Design review of the part built by this model. Coordinates are the model's own, in mm. A direction names the side the tool comes from. Give positions to 0.01 mm unless a question says otherwise; leave off trailing zeros. Order: outer loops, then holes, each group sorted by start corner. A loop starts at its lowest first (then second) coordinate and runs counter-clockwise, first axis right, second up. Notation, with made-up numbers: M 13.25,67 L 60.25,67 A15 cw 60.25,88 Z; hole C 60,40 d9. An arc over 180 degrees is marked long. Answer as a JSON object with one key per item and string values.
from build123d import *

# Parameters (mm, degrees)
SKETCH3_R          = 2.2
CUT_EXTRUDE1_DEPTH = 150


with BuildPart() as part:
    # Sketch1 → Revolve1 (revolve)
    with BuildSketch(Plane.XY, mode=Mode.PRIVATE) as revolve1_sk:
        with BuildLine():
            Line((0, 0), (152, 0))
            ThreePointArc((152, 0), (151.747967345, 2.795084972), (151, 5.5))
            Line((151, 5.5), (150, 5.5))
            Line((150, 5.5), (150, 4.5))
            Line((150, 4.5), (141, 4.5))
            Line((141, 4.5), (141, 3.5))
            Line((141, 3.5), (0, 3.5))
            Line((0, 3.5), (0, 0))
        make_face()
    revolve(revolve1_sk.sketch.rotate(Axis((0, 0, 0), (1, 0, 0)), 90), axis=Axis((0, 0, 0), (1, 0, 0)))

    # Sketch2 → Revolve2 (revolve)
    with BuildSketch(Plane.XY, mode=Mode.PRIVATE) as revolve2_sk:
        with BuildLine():
            Line((6, 0), (7, 0))
            Line((7, 0), (7, 3.5))
            ThreePointArc((7, 3.5), (6.5, 3.7), (6, 3.5))
            Line((6, 3.5), (6, 0))
        make_face()
    revolve(revolve2_sk.sketch.rotate(Axis((6, 0, 0), (1, 0, 0)), 90), axis=Axis((6, 0, 0), (1, 0, 0)))

    # Sketch3 → Cut-Extrude1 (cut)
    with BuildSketch(Plane.ZY):
        Circle(SKETCH3_R)
    extrude(amount=-CUT_EXTRUDE1_DEPTH, mode=Mode.SUBTRACT)


solid = part.part
(1) Insertion check: pin 1 (4 mm diameter, centred on x = 129, z = 0.5, fed in from -Y); pin 2 (6 mm diameter, centred on x = 109, z = 4, fed in from +Y); pin 3 (2.5 mm diameter, centred on y = 0, z = 0, fed in from -X). Each pin has a flat end and moves straight along its axis. Give the tip position at first contact, or say it passes through.
Checked values:
{"pin 1": "stops at y = -3.5", "pin 2": "stops at y = 3.35", "pin 3": "stops at x = 150"}
(2) We need section C-C (x = 70). Write out the cut boundary in (y, z).
Checked values:
{"outline": "C 0,0 d7; hole C 0,0 d4.4"}
(3) Draft analysis for pull direction Y (two halves, no side actions). For faces 1 (the cylindrical face through (73.062, 3.105, 1.615)), 2 (the cylindrical face through (73.95, 0.66, 2.1)), 3 (the flat face through (0, 2, -2)), state which applies: +Y half, -Y half, draft (parallel to the pull), parting line (faces both ways), or undercut.
Checked values:
{"face 1": "parting line", "face 2": "undercut", "face 3": "draft"}
(4) We need section A-A (y = 0). Write out the cut boundary in (x, z) (3 decimals).
Checked values:
{"outline": "M 0,-3.5 L 6,-3.5 A0.725 ccw 7,-3.5 L 141,-3.5 L 141,-4.5 L 150,-4.5 L 150,-5.5 L 151,-5.5 A15.625 ccw 151,5.5 L 150,5.5 L 150,4.5 L 141,4.5 L 141,3.5 L 7,3.5 A0.725 ccw 6,3.5 L 0,3.5 L 0,2.2 L 150,2.2 L 150,-2.2 L 0,-2.2 Z"}
(5) To check wall thickness, follow L1, parallel to Y at x = 76.5, z = 0; L2, parallel to Z at x = 55, y = 1.5; L3, parallel to Z at x = 10, y = 1.75. State the ranges of each line that lie inside material, in increasing order. Write a range as from..to.
Checked values:
{"L1": "y = -3.5..-2.2, 2.2..3.5", "L2": "z = -3.16..-1.61, 1.61..3.16", "L3": "z = -3.03..-1.33, 1.33..3.03"}
(6) Tool access review of faces 4 (the cylindrical face through (150.49, 5.37, -1.19)), 5 (the flat face through (150, 0, 0)), 6 (the flat face through (141, 4, 0)): name each direction out of +Z, -Z, +X, -X, +Y, -Y from which nothing blocks a thin tool from reaching the whole face with its end or side.
Checked values:
{"face 4": "+X, -X", "face 5": "-X", "face 6": "none"}
